```python
from build123d import *

# Parameters (mm, degrees)
F0_W        = 88.9
F0_H        = 165.1
F1_DEPTH    = 6.35
F2_DEPTH    = 25.4
F3_DEPTH    = 50.8
F4_C1_SIZE2 = 7.3323484187
F4_C1_SIZE  = 12.7
F4_C2_SIZE2 = 7.3323484187
F4_C2_SIZE  = 12.7
F4_C3_SIZE2 = 12.7
F4_C3_SIZE  = 7.3323484187
F4_C4_SIZE2 = 7.3323484187
F4_C4_SIZE  = 12.7
F5_C1_SIZE2 = 12.7
F5_C1_SIZE  = 7.3323484187
F5_C2_SIZE2 = 7.3323484187
F5_C2_SIZE  = 12.7
F5_C3_SIZE2 = 7.3323484187
F5_C3_SIZE  = 12.7
F5_C4_SIZE2 = 7.3323484187
F5_C4_SIZE  = 12.7
F6_R        = 6.34999


# Not quite as in the source:
# - a fillet or chamfer is up to 0.001 mm smaller than in the source, because OpenCascade refuses the exact size


with BuildPart() as f1:
    # F0 (on Top) → F1 (new body)
    with BuildSketch(Plane.XY):
        Rectangle(F0_W, F0_H)
        Polygon((0, 76.2), (38.1, 76.2), (38.1, -38.1), (38.1, -76.2), (0, -76.2), (-38.1, -76.2), (-38.1, 38.1), (-38.1, 76.2), align=None, mode=Mode.SUBTRACT)
    extrude(amount=F1_DEPTH)

    # F0 (on Top) → F2 (join)
    with BuildSketch(Plane.XY):
        with BuildLine():
            Line((38.1, -38.1), (38.1, 76.2))
            Line((38.1, 76.2), (0, 76.2))
            Line((0, 76.2), (0, 50.8))
            ThreePointArc((0, 50.8), (-3.7197438789, 41.8197438789), (-12.7, 38.1))
            Line((-12.7, 38.1), (-38.1, 38.1))
            Line((-38.1, 38.1), (-38.1, -76.2))
            Line((-38.1, -76.2), (0, -76.2))
            Line((0, -76.2), (0, -50.8))
            ThreePointArc((0, -50.8), (3.7197438789, -41.8197438789), (12.7, -38.1))
            Line((12.7, -38.1), (38.1, -38.1))
        make_face()
    extrude(amount=F2_DEPTH)

    # F0 (on Top) → F3 (join)
    with BuildSketch(Plane.XY):
        with BuildLine():
            Line((0, 50.8), (0, 76.2))
            Line((0, 76.2), (-38.1, 76.2))
            Line((-38.1, 76.2), (-38.1, 38.1))
            Line((-38.1, 38.1), (-12.7, 38.1))
            ThreePointArc((-12.7, 38.1), (-3.7197438789, 41.8197438789), (0, 50.8))
        make_face()
        with BuildLine():
            Line((38.1, -76.2), (38.1, -38.1))
            Line((38.1, -38.1), (12.7, -38.1))
            ThreePointArc((12.7, -38.1), (3.7197438789, -41.8197438789), (0, -50.8))
            Line((0, -50.8), (0, -76.2))
            Line((0, -76.2), (38.1, -76.2))
        make_face()
    extrude(amount=F3_DEPTH)

    # F4: chamfer of 12.7 x 7.3323484187 on 4 edges, made by hand

    # F4_c1
    f4_c1_edges = [f1.edges().sort_by_distance(p)[0] for p in [
        (-38.1, 57.15, 50.8),
    ]]
    f4_c1_side = f1.faces().sort_by_distance((-38.1, 57.15, 50.6533530316))[0]
    chamfer(f4_c1_edges, length=F4_C1_SIZE, length2=F4_C1_SIZE2, reference=f4_c1_side)

    # F4_c2
    f4_c2_edges = [f1.edges().sort_by_distance(p)[0] for p in [
        (-38.1, -19.05, 25.4),
    ]]
    f4_c2_side = f1.faces().sort_by_distance((-38.1, -19.05, 25.2533530316))[0]
    chamfer(f4_c2_edges, length=F4_C2_SIZE, length2=F4_C2_SIZE2, reference=f4_c2_side)

    # F4_c3
    f4_c3_edges = [f1.edges().sort_by_distance(p)[0] for p in [
        (-15.3838257906, -76.2, 25.4),
    ]]
    f4_c3_side = f1.faces().sort_by_distance((-15.3838257906, -76.2, 25.2533530316))[0]
    chamfer(f4_c3_edges, length=F4_C3_SIZE, length2=F4_C3_SIZE2, reference=f4_c3_side)

    # F4_c4
    f4_c4_edges = [f1.edges().sort_by_distance(p)[0] for p in [
        (-15.3838257906, 76.2, 50.8),
    ]]
    f4_c4_side = f1.faces().sort_by_distance((-15.3838257906, 76.2, 50.6533530316))[0]
    chamfer(f4_c4_edges, length=F4_C4_SIZE, length2=F4_C4_SIZE2, reference=f4_c4_side)

    # F5: chamfer of 12.7 x 7.3323484187 on 4 edges, made by hand

    # F5_c1
    f5_c1_edges = [f1.edges().sort_by_distance(p)[0] for p in [
        (19.05, 76.2, 25.4),
    ]]
    f5_c1_side = f1.faces().sort_by_distance((19.05, 76.2, 25.2533530316))[0]
    chamfer(f5_c1_edges, length=F5_C1_SIZE, length2=F5_C1_SIZE2, reference=f5_c1_side)

    # F5_c2
    f5_c2_edges = [f1.edges().sort_by_distance(p)[0] for p in [
        (38.1, 12.7, 25.4),
    ]]
    f5_c2_side = f1.faces().sort_by_distance((38.1, 12.7, 25.2533530316))[0]
    chamfer(f5_c2_edges, length=F5_C2_SIZE, length2=F5_C2_SIZE2, reference=f5_c2_side)

    # F5_c3
    f5_c3_edges = [f1.edges().sort_by_distance(p)[0] for p in [
        (38.1, -57.15, 50.8),
    ]]
    f5_c3_side = f1.faces().sort_by_distance((38.1, -57.15, 50.6533530316))[0]
    chamfer(f5_c3_edges, length=F5_C3_SIZE, length2=F5_C3_SIZE2, reference=f5_c3_side)

    # F5_c4
    f5_c4_edges = [f1.edges().sort_by_distance(p)[0] for p in [
        (15.3838257906, -76.2, 50.8),
    ]]
    f5_c4_side = f1.faces().sort_by_distance((15.3838257906, -76.2, 50.6533530316))[0]
    chamfer(f5_c4_edges, length=F5_C4_SIZE, length2=F5_C4_SIZE2, reference=f5_c4_side)

    # F6 (radius 6.35 in the source; OpenCascade refuses exactly that, so slightly less here)
    f6_edges = [f1.edges().sort_by_distance(p)[0] for p in [
        (-44.45, 0, 6.35),
        (0, -82.55, 6.35),
        (0, 82.55, 6.35),
        (44.45, 0, 6.35),
    ]]
    fillet(f6_edges, radius=F6_R)


solid = f1.part
```
Geometry: final body of the model. Coordinates: model frame, mm. A direction names the side the tool comes from. Round coordinates to 2 decimals unless told otherwise and drop trailing zeros. Loops run counter-clockwise (first coordinate to the right, second up) from the corner with the lowest first, then second, coordinate; pieces in that order, holes last.
Item 1: Line query: L1, parallel to Y at x = 31, z = 36; L2, parallel to Z at x = -15, y = -63; L3, parallel to Y at x = -32, z = 13. Output: solid intervals per line, ascending.
Checked values:
L1: y = -76.2 to -38.1
L2: z = 0 to 25.4
L3: y = -76.2 to 76.2
Item 2: Section B-B, the plane z = 42. Output: boundary loops of the cut face in (x, y), plus the area to 3 significant figures.
Checked values:
outline: (-35.85, 38.1) - (-12.7, 38.1) arc R12.7 ccw to (0, 50.8) - (0, 73.95) - (-35.85, 73.95) - close; (0, -73.95) - (35.85, -73.95) - (35.85, -38.1) - (12.7, -38.1) arc R12.7 ccw to (0, -50.8) - close
area: 2,500 mm2
Item 3: Section D-D, the plane z = 16. Output: boundary loops of the cut face in (x, y).
Checked values:
outline: (-38.1, 38.1) - (-36.19, 38.1) - (-36.19, -76.2) - (38.1, -76.2) - (38.1, -38.1) - (36.19, -38.1) - (36.19, 76.2) - (-38.1, 76.2) - close
Item 4: Reachability of faces 1 (the flat face through (0, 63, 38)), 2 (the flat face through (-17.745, -69.761, 21.785)), 3 (the flat face through (-8, 76.2, 18)), 4 (the flat face through (38.1, -35, 11)) from +Z, -Z, +X, -X, +Y, -Y: full face, straight path, thin tool, end or side. Return the list, or none.
Checked values:
face 1: +Z, +X, +Y
face 2: +Z, -X, -Y
face 3: +Z, +X, -X, +Y
face 4: +Z, +X, +Y, -Y
Item 5: Contact query for flat-ended pins moving along their axis: P1, Ø8, axis at x = 2, y = -24.5, coming from the +Z side; P2, Ø4, axis at y = 45.5, z = 35.5, coming from the +X side; P3, Ø8, axis at x = -22.5, z = 13, coming from the -Y side; P4, Ø8, axis at x = -9.5, y = 13, coming from the -Z side. Output: stop coordinate, or through.
Checked values:
P1: stops at z = 25.4
P2: stops at x = -0.44
P3: stops at y = -76.2
P4: stops at z = 0
